Input: part model. Units: mm. Frame: model coordinates. Face numbers are marked on the shaded views. A direction names the side the tool comes from. Give positions to 0.01 mm unless a question says otherwise; leave off trailing zeros. Loops run counter-clockwise (first coordinate to the right, second up) from the corner with the lowest first, then second, coordinate; pieces in that order, holes last. Notation, with made-up numbers: (-8, -12.75) -> (37, -12.75) arc R17 cw to (37, 6.25) -> close; hole circle Ø5 at (2, -8). An arc over 180 degrees is marked (long way). One line per question, with ' | ' between items.
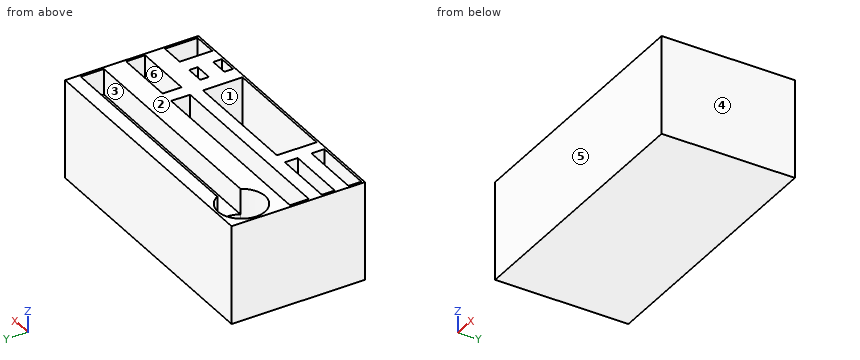
from build123d import *

# Parameters (mm, degrees)
F0_W      = 315
F0_H      = 155
F1_DEPTH  = 115
F3_W      = 225
F3_H      = 22
F9_DEPTH  = 100
F10_DEPTH = 55
F11_DEPTH = 30
F4_W      = 70
F4_H      = 15
F12_DEPTH = 80
F5_W      = 140
F5_H      = 46
F13_DEPTH = 100
F6_W      = 69
F6_H      = 22
F14_DEPTH = 100
F7_W      = 21
F7_H      = 10
F15_DEPTH = 35
F8_W      = 28
F8_H      = 38
F16_DEPTH = 25


with BuildPart() as f1:
    # F0 (on Top) → F1 (new body)
    with BuildSketch(Plane.XY):
        Rectangle(F0_W, F0_H)
    extrude(amount=-F1_DEPTH)

    # F3 (on face) → F9 (cut)
    with BuildSketch(Plane.XY):
        with Locations((-42.5, -3)):
            Rectangle(F3_W, F3_H)
    extrude(amount=-F9_DEPTH, mode=Mode.SUBTRACT)

    # F2 (on face) → F10 (cut)
    with BuildSketch(Plane.XY):
        with BuildLine():
            ThreePointArc((-103.541703, 34), (-100.900158, 40.521575), (-100, 47.5))
            ThreePointArc((-100, 47.5), (-100.900158, 54.478425), (-103.541703, 61))
            ThreePointArc((-103.541703, 61), (-155, 47.5), (-103.541703, 34))
        make_face()
    extrude(amount=-F10_DEPTH, mode=Mode.SUBTRACT)

    # F4 (on face) → F11 (cut)
    with BuildSketch(Plane.XY):
        with BuildLine():
            ThreePointArc((-103.541703, 61), (-155, 47.5), (-103.541703, 34))
            Line((-103.541703, 34), (155, 34))
            Line((155, 34), (155, 61))
            Line((155, 61), (-103.541703, 61))
        make_face()
    extrude(amount=-F11_DEPTH, mode=Mode.SUBTRACT)

    # F4 (on face) → F12 (cut)
    with BuildSketch(Plane.XY):
        with Locations((-120, -36.5)):
            Rectangle(F4_W, F4_H)
        with Locations((-120, -67.5)):
            Rectangle(F4_W, F4_H)
    extrude(amount=-F12_DEPTH, mode=Mode.SUBTRACT)

    # F5 (on face) → F13 (cut)
    with BuildSketch(Plane.XY):
        with Locations((0, -52)):
            Rectangle(F5_W, F5_H)
    extrude(amount=-F13_DEPTH, mode=Mode.SUBTRACT)

    # F6 (on face) → F14 (cut)
    with BuildSketch(Plane.XY):
        with Locations((120.5, -3)):
            Rectangle(F6_W, F6_H)
    extrude(amount=-F14_DEPTH, mode=Mode.SUBTRACT)

    # F7 (on face) → F15 (cut)
    with BuildSketch(Plane.XY):
        with Locations((98.5, -42)):
            Rectangle(F7_W, F7_H)
        with Locations((98.5, -70)):
            Rectangle(F7_W, F7_H)
    extrude(amount=-F15_DEPTH, mode=Mode.SUBTRACT)

    # F8 (on face) → F16 (cut)
    with BuildSketch(Plane.XY):
        with Locations((141, -56)):
            Rectangle(F8_W, F8_H)
    extrude(amount=-F16_DEPTH, mode=Mode.SUBTRACT)


solid = f1.part
1. Pull-direction query (Y, two-part tool) for the marked faces 3, 4, 5 and 6; classes: pulls with the +Y half, pulls with the -Y half, needs draft (parallel to the pull), parting line crosses it, or undercut.
Determined:
face 3: undercut | face 4: needs draft | face 5: pulls with the -Y half | face 6: undercut
2. Section query D-D (y = -40). Output: boundary loops of the cut face in (x, z).
Determined:
outline: (-157.5, -115) -> (157.5, -115) -> (157.5, 0) -> (155, 0) -> (155, -25) -> (127, -25) -> (127, 0) -> (109, 0) -> (109, -35) -> (88, -35) -> (88, 0) -> (70, 0) -> (70, -100) -> (-70, -100) -> (-70, 0) -> (-85, 0) -> (-85, -80) -> (-155, -80) -> (-155, 0) -> (-157.5, 0) -> close
3. Section query C-C (z = -88). Output: boundary loops of the cut face in (x, y).
Determined:
outline: (-157.5, -77.5) -> (157.5, -77.5) -> (157.5, 77.5) -> (-157.5, 77.5) -> close; hole (-155, -14) -> (70, -14) -> (70, 8) -> (-155, 8) -> close; hole (-70, -75) -> (70, -75) -> (70, -29) -> (-70, -29) -> close; hole (86, -14) -> (155, -14) -> (155, 8) -> (86, 8) -> close
4. Section query A-A (z = -62). Output: boundary loops of the cut face in (x, y), then the cut area to 3 significant figures.
Determined:
outline: (-157.5, -77.5) -> (157.5, -77.5) -> (157.5, 77.5) -> (-157.5, 77.5) -> close; hole (-155, -75) -> (-85, -75) -> (-85, -60) -> (-155, -60) -> close; hole (-155, -44) -> (-85, -44) -> (-85, -29) -> (-155, -29) -> close; hole (-155, -14) -> (70, -14) -> (70, 8) -> (-155, 8) -> close; hole (-70, -75) -> (70, -75) -> (70, -29) -> (-70, -29) -> close; hole (86, -14) -> (155, -14) -> (155, 8) -> (86, 8) -> close | area: 33,800 mm2
5. Reachability of the marked faces 1 and 2 from +Z, -Z, +X, -X, +Y, -Y: full face, straight path, thin tool, end or side. Return the list, or none.
Determined:
face 1: +Z | face 2: +Z, +X, -X, +Y, -Y
6. Section query B-B (x = -63.5). Output: boundary loops of the cut face in (y, z).
Determined:
outline: (-77.5, -115) -> (77.5, -115) -> (77.5, 0) -> (61, 0) -> (61, -30) -> (34, -30) -> (34, 0) -> (8, 0) -> (8, -100) -> (-14, -100) -> (-14, 0) -> (-29, 0) -> (-29, -100) -> (-75, -100) -> (-75, 0) -> (-77.5, 0) -> close
7. Ray query, line 1 along Y through (x, z) = (-127.5, -17); line 2 along Y through (x, z) = (39.5, -51); line 3 along X through (y, z) = (-54, -23). Return the intervals inside material, ascending. Write a range as from..to.
Determined:
line 1: y = -77.5..-75, -60..-44, -29..-14, 8..20, 75..77.5 | line 2: y = -77.5..-75, -29..-14, 8..77.5 | line 3: x = -157.5..-70, 70..127, 155..157.5
8. Pin query (flat end, axial travel): P1, Ø6, axis at x = 115, y = 3, coming from the +Z side; P2, Ø5, axis at x = 101.5, y = -71.5, coming from the +Z side. Return the tip coordinate at first contact, or that it passes through.
Determined:
P1: stops at z = -100 | P2: stops at z = -35
